Geometry check sheet. Reference: the model listing, model coordinates, mm. Coordinates: 2 decimals unless noted, no trailing zeros. Write each loop counter-clockwise with the first axis right and the second up, starting at its lowest first coordinate (ties: lowest second). Pieces come first, ordered by that corner, then holes. Notation, with made-up numbers: M 44.5,-6 L 100.5,-6 A16 ccw 100.5,14 Z; hole C 50,-11.5 d3. An arc over 180 degrees is marked long. Write item = value, one per line. Start each with the question number.
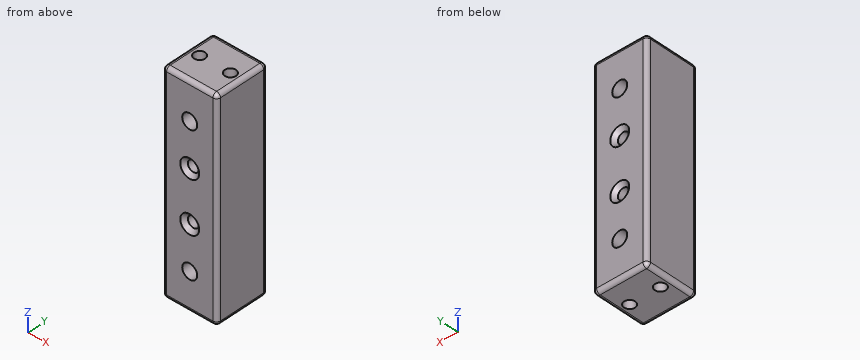
```python
from build123d import *

# Parameters (mm, degrees)
SKETCH1_W           = 13.75
SKETCH1_H           = 13.75
BOSS_EXTRUDE1_DEPTH = 54
SKETCH3_R           = 1.9
SKETCH3_R_2         = 1.4
CUT_EXTRUDE2_DEPTH  = 57.145597557
SKETCH9_R           = 1.4
CUT_EXTRUDE7_DEPTH  = 55.868308248
FILLET2_R           = 1
CHAMFER1_SIZE       = 1


with BuildPart() as part:
    # Sketch1 → Boss-Extrude1 (new body)
    with BuildSketch(Plane.XY):
        Rectangle(SKETCH1_W, SKETCH1_H)
    extrude(amount=BOSS_EXTRUDE1_DEPTH)

    # Sketch3 → Cut-Extrude2 (cut, through all)
    with BuildSketch(Plane(origin=(0, 6.875, 0), x_dir=(1, 0, 0), z_dir=(0, 1, 0))):
        with Locations(Location((0, -9.5, 0), (0, 0, 270))):
            Circle(SKETCH3_R)
        with Locations(Location((0, -44.5, 0), (0, 0, 270))):
            Circle(SKETCH3_R)
        with Locations(Location((0, -20.5, 0), (0, 0, 270))):
            Circle(SKETCH3_R_2)
        with Locations(Location((0, -33.5, 0), (0, 0, 270))):
            Circle(SKETCH3_R_2)
    extrude(amount=-CUT_EXTRUDE2_DEPTH, mode=Mode.SUBTRACT)

    # Sketch9 → Cut-Extrude7 (cut, through all)
    with BuildSketch(Plane(origin=(0, 0, 0), x_dir=(-1, 0, 0), z_dir=(0, 0, -1))):
        with Locations((-3.9, 0)):
            Circle(SKETCH9_R)
    cut_extrude7 = extrude(amount=-CUT_EXTRUDE7_DEPTH, mode=Mode.SUBTRACT)

    # Mirror5: Cut-Extrude7 across plane
    add(cut_extrude7.mirror(Plane(origin=(0, 0, 0), x_dir=(0, 0, 1), z_dir=(1, 0, 0))), mode=Mode.SUBTRACT)

    # Fillet2
    fillet2_edges = [part.edges().sort_by_distance(p)[0] for p in [
        (-6.875, 0, 54),
        (0, -6.875, 54),
        (6.875, 0, 54),
        (0, -6.875, 0),
        (-6.875, 0, 0),
        (0, 6.875, 0),
        (6.875, 0, 0),
        (6.875, -6.875, 27),
        (-6.875, -6.875, 27),
        (-6.875, 6.875, 27),
        (6.875, 6.875, 27),
        (0, 6.875, 54),
    ]]
    fillet(fillet2_edges, radius=FILLET2_R)

    # Chamfer1
    chamfer1_edges = [part.edges().sort_by_distance(p)[0] for p in [
        (0, -6.875, 32.1),
        (0, 6.875, 32.1),
        (0, -6.875, 19.1),
        (0, 6.875, 19.1),
    ]]
    chamfer(chamfer1_edges, length=CHAMFER1_SIZE)


solid = part.part
```
Q1. Cross-section at D-D on z = 24. Enter the section's corners in (x, y) (3 decimals), and give its area (3 significant figures).
Q2. Scan lines: L1, parallel to Y at x = -3.9, z = 27 (3 decimals); L2, parallel to Z at x = -0.5, y = -1.5. Record each from-to range of solid material in increasing order.
Q3. Cross-section at B-B on z = 9.5. Enter the section's corners in (x, y) (3 decimals).
Q4. Cross-section at C-C on x = -3.9. Enter the section's corners in (y, z) (3 decimals).
Q5. Gauge pin test, flat ends, axial feed: pin 1 (2.5 mm diameter, centred on x = 0, z = 33.5, fed in from +Y); pin 2 (3 mm diameter, centred on x = 0, z = 20.5, fed in from -Y) (3 decimals). Record the tip position at first contact, or that the pin passes through.
Q6. Cross-section at A-A on y = 0. Enter the section's corners in (x, z) (3 decimals).
Values found:
q1.outline = M -6.875,-5.875 A1 ccw -5.875,-6.875 L 5.875,-6.875 A1 ccw 6.875,-5.875 L 6.875,5.875 A1 ccw 5.875,6.875 L -5.875,6.875 A1 ccw -6.875,5.875 Z; hole C -3.9,0 d2.8; hole C 3.9,0 d2.8
q1.area = 176 mm²
q2.L1 = -6.875 to -1.4, 1.4 to 6.875
q2.L2 = 0 to 7.67, 11.33 to 19.19, 21.81 to 32.19, 34.81 to 42.67, 46.33 to 54
q3.outline = M -6.875,-5.875 A1 ccw -5.875,-6.875 L -1.9,-6.875 L -1.9,6.875 L -5.875,6.875 A1 ccw -6.875,5.875 Z; M 1.9,-6.875 L 5.875,-6.875 A1 ccw 6.875,-5.875 L 6.875,5.875 A1 ccw 5.875,6.875 L 1.9,6.875 Z; hole C -3.9,0 d2.8; hole C 3.9,0 d2.8
q4.outline = M -6.875,1 A1 ccw -5.875,0 L -1.4,0 L -1.4,54 L -5.875,54 A1 ccw -6.875,53 Z; M 1.4,0 L 5.875,0 A1 ccw 6.875,1 L 6.875,53 A1 ccw 5.875,54 L 1.4,54 Z
q5.pin_1 = through
q5.pin_2 = -5.975
q6.outline = M -6.875,1 A1 ccw -5.875,0 L -5.3,0 L -5.3,54 L -5.875,54 A1 ccw -6.875,53 Z; M -2.5,0 L 2.5,0 L 2.5,54 L -2.5,54 Z; M 5.3,0 L 5.875,0 A1 ccw 6.875,1 L 6.875,53 A1 ccw 5.875,54 L 5.3,54 Z; hole C 0,9.5 d3.8; hole C 0,44.5 d3.8; hole C 0,20.5 d2.8; hole C 0,33.5 d2.8
